Source: CAD feature listing. Evaluate the final solid. Frame: model axes, mm. Face numbers are marked on the shaded views. A direction names the side the tool comes from. Give positions to 0.01 mm unless a question says otherwise; leave off trailing zeros. Order: outer loops, then holes, each group sorted by start corner. A loop starts at its lowest first (then second) coordinate and runs counter-clockwise, first axis right, second up. Notation, with made-up numbers: M 4,82 L 20,82 A9 cw 20,89 Z; hole C 45.25,8 d4. An arc over 180 degrees is marked long. Answer as a JSON object with one key per item and string values. Group by question number.
1. Set-up query: the marked faces 1 and 2. Return all of +Z, -Z, +X, -X, +Y, -Y with unobstructed straight access to the full face (end or side cutting, diameter ignored); none if empty.
2. Section query B-B (y = -32). Output: boundary loops of the cut face in (x, z), plus the area to 3 significant figures.
3. Pull-direction query (Y, two-part tool) for the marked faces 3, 4 and 5; classes: +Y half, -Y half, draft (parallel to the pull), parting line (faces both ways), or undercut.
4. Section query C-C (x = 4.5). Output: boundary loops of the cut face in (y, z), plus the area to 3 significant figures.
5. Pin query (flat end, axial travel): P1, Ø1.5, axis at y = -3.5, z = 1.5, coming from the +X side; P2, Ø2.5, axis at y = -38.5, z = -3, coming from the -X side; P3, Ø7, axis at x = 33.5, z = 3, coming from the +Y side. Return the tip coordinate at first contact, or that it passes through.
6. Section query D-D (x = 21). Output: boundary loops of the cut face in (y, z), plus the area to 3 significant figures.
7. Material intervals for L1, parallel to Y at x = 5.5, z = -4.75; L2, parallel to X at y = -31, z = 10; L3, parallel to Z at x = 24.5, y = -42.5, sorted ascending. Write a range as [from, to].
8. Section query A-A (z = -5). Output: boundary loops of the cut face in (x, y).
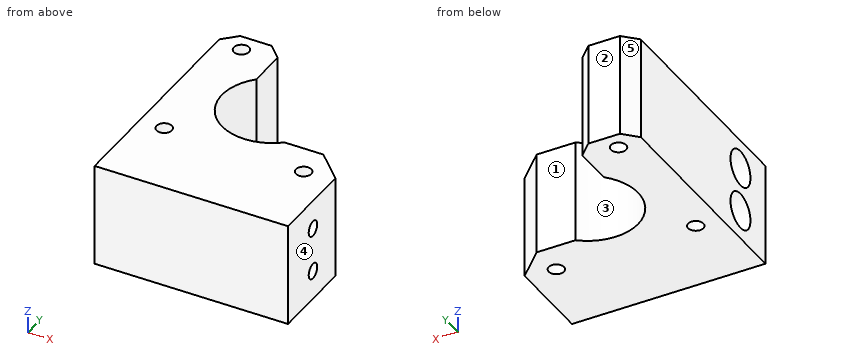
Autodesk Inventor part; units mm, degrees
ref_plane "YZ Plane" through (0, 0, 0) normal (1, 0, 0) x (0, 1, 0)
ref_plane "XZ Plane" through (0, 0, 0) normal (0, 1, 0) x (-1, 0, 0)
ref_plane "XY Plane" through (0, 0, 0) normal (0, 0, 1) x (1, 0, 0)
sketch "Sketch1" plane through (0, 0, 0) normal (0, 0, 1) x (1, 0, 0)
  line L0 (0, 0) -> (3, 3)
  line L1 (3, 3) -> (10, 3)
  line L2 (10, 3) -> (13, 0)
  line L3 (13, 0) -> (13, -8.5904)
  circle A0 centre (21, -16.5) radius 11.25
  line L4 (28.3697, -25) -> (37, -25)
  line L5 (37, -25) -> (43, -31)
  line L6 (43, -31) -> (43, -50)
  line L7 (43, -50) -> (0, -50)
  line L8 (0, -50) -> (0, 0)
  circle A1 centre (5.5, -1) radius 1.7
  circle A2 centre (5.5, -32) radius 1.7
  circle A3 centre (36.5, -32) radius 1.7
  line L9 (5.5, -32) -> (5.5, -1) construction
  line L10 (5.5, -32) -> (36.5, -32) construction
  dimension "d0" = 16.5
  dimension "d1" = 21
  dimension "d2" = 50
  dimension "d3" = 22.5
  dimension "d4" = 8
  dimension "d5" = 45
  dimension "d6" = 3
  dimension "d7" = 8.5
  dimension "d8" = 6
  dimension "d11" = 22
  dimension "d14" = 3.4
  dimension "d15" = 15.5
  dimension "d16" = 31
  dimension "d17" = 31
  dimension "d18" = 15.5
extrude "Extrusion1" add sketch "Sketch1" along normal mid plane 23 contours L0 L1 L2 L3 A0 L4 L5 L6 L7 L8
sketch "Sketch2" plane through (0, -50, 11.5) normal (-1, 0, 0) x (0, 0, 1)
  line L0 (-23, 53) -> (0, 53) construction
  line L1 (-11.5, 53) -> (-11.5, 0) construction
  line L2 (-23, 0) -> (0, 0) construction
  circle A0 centre (-16.5, 10) radius 1.7
  circle A1 centre (-6.5, 10) radius 1.7
  point P0 (-11.5, 50)
  dimension "d22" = 10
  dimension "d23" = 10
  dimension "d24" = 3.4
extrude "Extrusion2" cut sketch "Sketch2" against normal through all
sketch "Sketch3" plane through (0, -50, 11.5) normal (-1, 0, 0) x (0, 0, 1)
  circle A0 centre (-16.5, 10) radius 1.7
  circle A1 centre (-16.5, 10) radius 4
  circle A2 centre (-6.5, 10) radius 1.7
  circle A3 centre (-6.5, 10) radius 4
  point P0 (-11.5, 50)
  dimension "d27" = 8
  dimension "d28" = 8
extrude "Extrusion3" cut sketch "Sketch3" against normal blind 35 contours A0 | A1 | A2 | A3
equation "\"d17\" = d16"
properties part number "y-stepper-mount"
Answer sheet:
{
 "1": {"face 1": "+Z, -Z, +X, +Y", "face 2": "+Z, -Z, +X, -X, +Y"},
 "2": {"outline": "M 0,-11.5 L 3.8,-11.5 L 3.8,11.5 L 0,11.5 Z; M 7.2,-11.5 L 34.8,-11.5 L 34.8,11.5 L 7.2,11.5 Z; M 38.2,-11.5 L 43,-11.5 L 43,11.5 L 38.2,11.5 Z", "area": "833 mm^2"},
 "3": {"face 3": "undercut", "face 4": "draft", "face 5": "+Y half"},
 "4": {"outline": "M -50,-11.5 L -33.37,-11.5 L -33.37,11.5 L -50,11.5 Z; M -30.63,-11.5 L -2.37,-11.5 L -2.37,11.5 L -30.63,11.5 Z; M 0.37,-11.5 L 3,-11.5 L 3,11.5 L 0.37,11.5 Z; hole C -40,-5 d8; hole C -40,5 d8", "area": "992 mm^2"},
 "5": {"P1": "x = 13", "P2": "x = 35", "P3": "y = -25"},
 "6": {"outline": "M -50,-11.5 L -27.75,-11.5 L -27.75,11.5 L -50,11.5 Z; hole C -40,-5 d8; hole C -40,5 d8", "area": "411 mm^2"},
 "7": {"L1": "[-50, -43.99], [-36.01, -33.7], [-30.3, -2.7], [0.7, 3]", "L2": "[0, 4.13], [6.87, 35.13], [37.87, 43]", "L3": "[-11.5, -8.12], [-1.88, 1.88], [8.12, 11.5]"},
 "8": {"outline": "M 0,-50 L 43,-50 L 43,-41.7 L 35,-41.7 L 35,-44 L 0,-44 Z; M 0,-36 L 35,-36 L 35,-38.3 L 43,-38.3 L 43,-31 L 37,-25 L 28.37,-25 A11.25 cw 13,-8.59 L 13,0 L 10,3 L 3,3 L 0,0 Z; hole C 5.5,-32 d3.4; hole C 5.5,-1 d3.4; hole C 36.5,-32 d3.4"}
}
